Geometry check sheet. Reference: drawing and pictorial views, mm from the part's lowest x, y, z. Round coordinates to 2 decimals unless told otherwise and drop trailing zeros. Write each loop counter-clockwise with the first axis right and the second up, starting at its lowest first coordinate (ties: lowest second). Pieces come first, ordered by that corner, then holes. Notation, with made-up numbers: M 57,49.5 L 65,49.5 A14 ccw 65,53.5 Z; hole C -15.5,77.5 d9. An arc over 180 degrees is marked long. One line per item, written item: value. Start each with the question number.
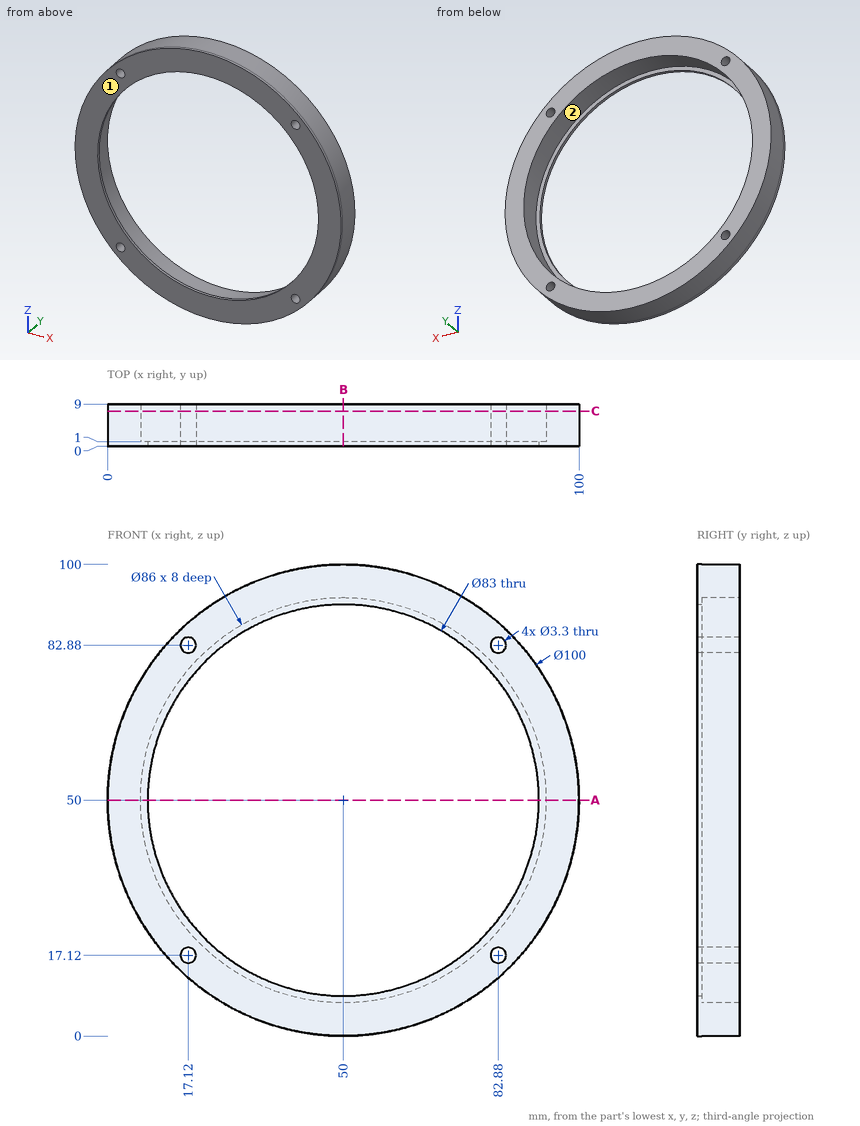
1) Mould release check, pull along X, two halves, no side actions. Record for the marked faces 1 and 2: pulls with the +X half, pulls with the -X half, needs draft (parallel to the pull), parting line crosses it, or undercut.
2) Cross-section at C-C (y = 7.5). Record the boundary of the cut face in (x, z).
3) Thickness scan on line 1 (X direction, y = 0.25, z = 50); line 2 (X direction, y = 5.5, z = 50); line 3 (Z direction, x = 34, y = 1.75). Record the ranges inside material, lowest first.
4) Gauge pin test, flat ends, axial feed: pin 1 Ø5 at (y, z) = (1, 71.5) entering from -X; pin 2 Ø2 at (x, y) = (74.5, 7) entering from -Z; pin 3 Ø1.5 at (x, y) = (65.5, 7.5) entering from -Z (1 decimal); pin 4 Ø5.5 at (x, z) = (82.88, 82.88) entering from +Y. Record the tip position at first contact, or that the pin passes through.
5) Cross-section at A-A (z = 50). Record the boundary of the cut face in (x, y), then the cut area to 3 significant figures.
6) Cross-section at B-B (x = 50). Record the boundary of the cut face in (y, z), then the cut area to 3 significant figures.
Results below:
1. face 1: needs draft
1. face 2: undercut
2. outline: C 50,50 d100; hole C 50,50 d86; hole C 17.12,17.12 d3.3; hole C 17.12,82.88 d3.3; hole C 82.88,17.12 d3.3; hole C 82.88,82.88 d3.3
3. line 1: x = 0 to 8.5, 91.5 to 100
3. line 2: x = 0 to 7, 93 to 100
3. line 3: z = 2.63 to 10.09, 89.91 to 97.37
4. pin 1: stops at x = 3.75
4. pin 2: stops at z = 5.87
4. pin 3: stops at z = 2.2
4. pin 4: stops at y = 9
5. outline: M 0,0 L 8.5,0 L 8.5,1 L 7,1 L 7,9 L 0,9 Z; M 91.5,0 L 100,0 L 100,9 L 93,9 L 93,1 L 91.5,1 Z
5. area: 129 mm²
6. outline: M 0,0 L 9,0 L 9,7 L 1,7 L 1,8.5 L 0,8.5 Z; M 0,91.5 L 1,91.5 L 1,93 L 9,93 L 9,100 L 0,100 Z
6. area: 129 mm²
